Solid Edge part; units mm, degrees
sketch "Sketch1" plane through (0, 0, 0) normal (0, 0, 1) x (1, 0, 0)
  circle A0 centre (0, 0) radius 5
extrude "Protrusion1" add sketch "Sketch1" along normal mid plane 20
chamfer "Chamfer1" distance 0.75 angle 45 2 edges at (-5, 0, -10) (-5, 0, 10)
sketch "Sketch2" plane through (0, 0, 10) normal (0, 0, 1) x (1, 0, 0)
  line L0 (-1.4434, 2.5) -> (1.4434, 2.5)
  line L1 (2.8868, 0) -> (1.4434, 2.5)
  line L2 (1.4434, -2.5) -> (2.8868, 0)
  line L3 (-1.4434, -2.5) -> (1.4434, -2.5)
  line L4 (-2.8868, 0) -> (-1.4434, -2.5)
  line L5 (-1.4434, 2.5) -> (-2.8868, 0)
extrude "Cutout1" cut sketch "Sketch2" against normal blind 10
properties part number "24104618"
Geometry check sheet. Reference: the model listing, model coordinates, mm. A direction names the side the tool comes from. Coordinates: 2 decimals unless noted, no trailing zeros. Order: outer loops, then holes, each group sorted by start corner. A loop starts at its lowest first (then second) coordinate and runs counter-clockwise, first axis right, second up.
Item 1: Section check C-C (z = -0.25). Enter the section's corners in (x, y), plus the area to 3 significant figures.
Item 2: Tool access check on faces 4 (the flat face through (0, 2.5, 5)), 5 (the flat face through (-2, -2, 10)). Record the directions out of +Z, -Z, +X, -X, +Y, -Y that give a thin tool (end or side, any length) a straight path to the whole face; none if there is none.
Item 3: Depth check by flat-ended pin: pin 1 (1.5 mm diameter, centred on y = -3.5, z = -5.5, fed in from -X); pin 2 (1 mm diameter, centred on y = -1, z = 0, fed in from -X); pin 3 (1.5 mm diameter, centred on x = -0.5, y = 0, fed in from +Z). Enter the tip coordinate at first touch or a pass-through.
Item 4: Mould release check, pull along X, two halves, no side actions. Record for faces 1 (the flat face through (0, 0, -10)), 2 (the flat face through (0, 0, 0)), 3 (the cylindrical face through (-1.08, -4.88, 0.13)): released by +X, released by -X, zero draft, split by the parting line, or undercut.
Item 5: Section check A-A (z = 8.5). Enter the section's corners in (x, y), plus the area to 3 significant figures.
Item 6: Scan lines: line 1 along Z through (x, y) = (0.5, -1.5); line 2 along Y through (x, z) = (-0.75, 7); line 3 along Y through (x, z) = (1.5, 2.75). Record each from-to range of solid material in increasing order.
Item 7: Section check B-B (x = 0). Enter the section's corners in (y, z).
Check sheet entries:
1. outline: circle Ø10 at (0, 0)
1. area: 78.5 mm2
2. face 4: +Z
2. face 5: +Z, +X, -X, +Y, -Y
3. pin 1: stops at x = -4.18
3. pin 2: stops at x = -4.97
3. pin 3: stops at z = 0
4. face 1: zero draft
4. face 2: undercut
4. face 3: split by the parting line
5. outline: circle Ø10 at (0, 0); hole (-2.89, 0) - (-1.44, -2.5) - (1.44, -2.5) - (2.89, 0) - (1.44, 2.5) - (-1.44, 2.5) - close
5. area: 56.9 mm2
6. line 1: z = -10 to 0
6. line 2: y = -4.94 to -2.5, 2.5 to 4.94
6. line 3: y = -4.77 to -2.4, 2.4 to 4.77
7. outline: (-5, -9.25) - (-4.25, -10) - (4.25, -10) - (5, -9.25) - (5, 9.25) - (4.25, 10) - (2.5, 10) - (2.5, 0) - (-2.5, 0) - (-2.5, 10) - (-4.25, 10) - (-5, 9.25) - close
